Drawing for the job (mm, zero at the part's lowest x, y, z). Coordinates: 2 decimals unless noted, no trailing zeros. Write each loop counter-clockwise with the first axis right and the second up, starting at its lowest first coordinate (ties: lowest second). Pieces come first, ordered by that corner, then holes. Notation, with made-up numbers: (23, 19.5) -> (44, 19.5) arc R18 cw to (44, 25.5) -> close; hole circle Ø4 at (-0.75, 59). An arc over 180 degrees is marked (long way). Answer as CSV lines item,"result".
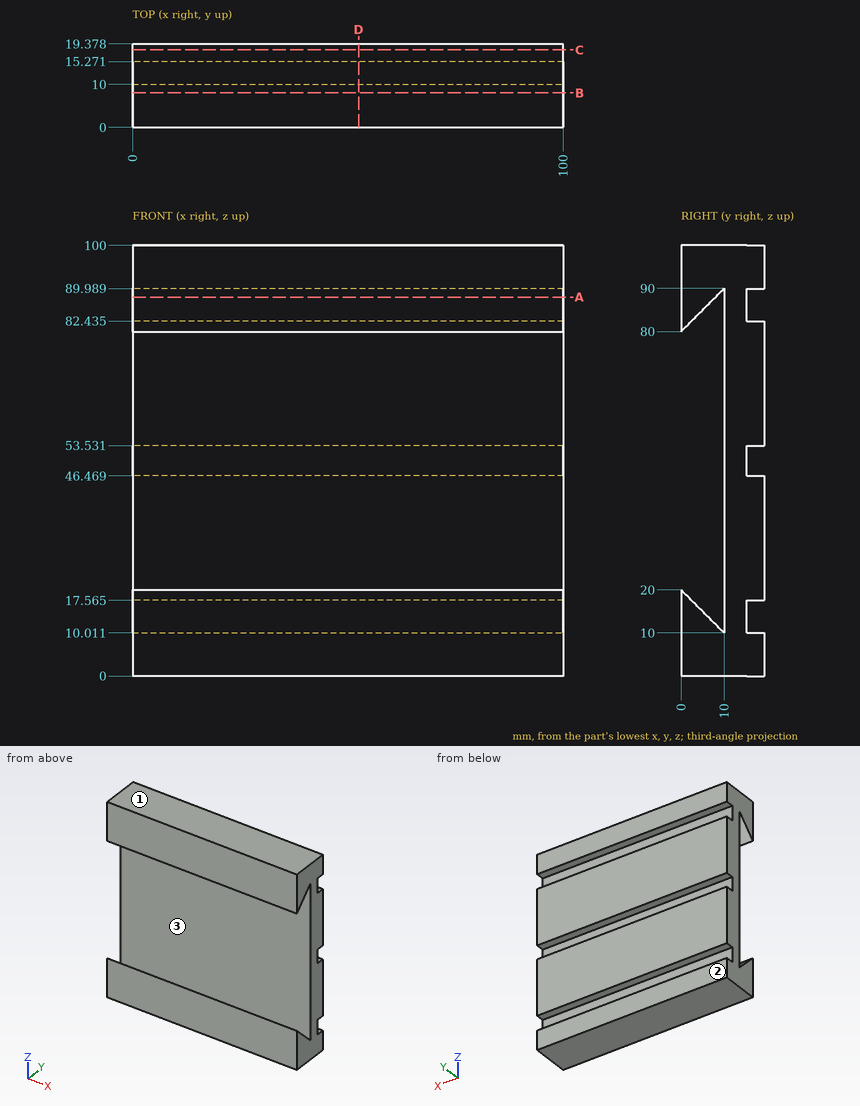
Item 1: Flat gauge pins, fed straight in: pin 1 (2 mm diameter, centred on x = 71, z = 48.5, fed in from +Y); pin 2 (12 mm diameter, centred on x = 50.5, z = 61.5, fed in from -Y). Where does each tip first touch, or does it go through?
Answer below:
pin 1,"stops at y = 15.27"
pin 2,"stops at y = 10"
Item 2: Saw through at B-B on y = 8. Give the cut face in (x, z), and give its area (3 significant figures).
Answer below:
outline,"(0, 0) -> (100, 0) -> (100, 12) -> (0, 12) -> close; (0, 88) -> (100, 88) -> (100, 100) -> (0, 100) -> close"
area,"2,400 mm2"
Item 3: Saw through at A-A on z = 88. Give the cut face in (x, y).
Answer below:
outline,"(0, 0) -> (100, 0) -> (100, 8) -> (0, 8) -> close; (0, 10) -> (100, 10) -> (100, 15.27) -> (0, 15.27) -> close"
Item 4: Saw through at D-D on x = 52.5. Give the cut face in (y, z) (1 decimal).
Answer below:
outline,"(0, 0) -> (19.4, 0) -> (19.4, 10) -> (15.3, 10) -> (15.3, 17.6) -> (19.4, 17.6) -> (19.4, 46.5) -> (15.3, 46.5) -> (15.3, 53.5) -> (19.4, 53.5) -> (19.4, 82.4) -> (15.3, 82.4) -> (15.3, 90) -> (19.4, 90) -> (19.4, 100) -> (0, 100) -> (0, 80) -> (10, 90) -> (10, 10) -> (0, 20) -> close"
Item 5: Wall check: line 1 (Z direction, x = 37.5, y = 17.5) (1 decimal); line 2 (Y direction, x = 71, z = 36); line 3 (Y direction, x = 8, z = 50). Give the ranges that are in metal, low to high. Write a range as from..to.
Answer below:
line 1,"z = 0..10, 17.6..46.5, 53.5..82.4, 90..100"
line 2,"y = 10..19.38"
line 3,"y = 10..15.27"
Item 6: Two-plate mould, pull along Z, no slides. Class the marked faces 1, 2 and 3: pulls with the +Z half, pulls with the -Z half, needs draft (parallel to the pull), parting line crosses it, or undercut.
Answer below:
face 1,"pulls with the +Z half"
face 2,"needs draft"
face 3,"undercut"
Item 7: Saw through at C-C on y = 18. Give the cut face in (x, z) (1 decimal), and give its area (3 significant figures).
Answer below:
outline,"(0, 0) -> (100, 0) -> (100, 10) -> (0, 10) -> close; (0, 17.6) -> (100, 17.6) -> (100, 46.5) -> (0, 46.5) -> close; (0, 53.5) -> (100, 53.5) -> (100, 82.4) -> (0, 82.4) -> close; (0, 90) -> (100, 90) -> (100, 100) -> (0, 100) -> close"
area,"7,780 mm2"
